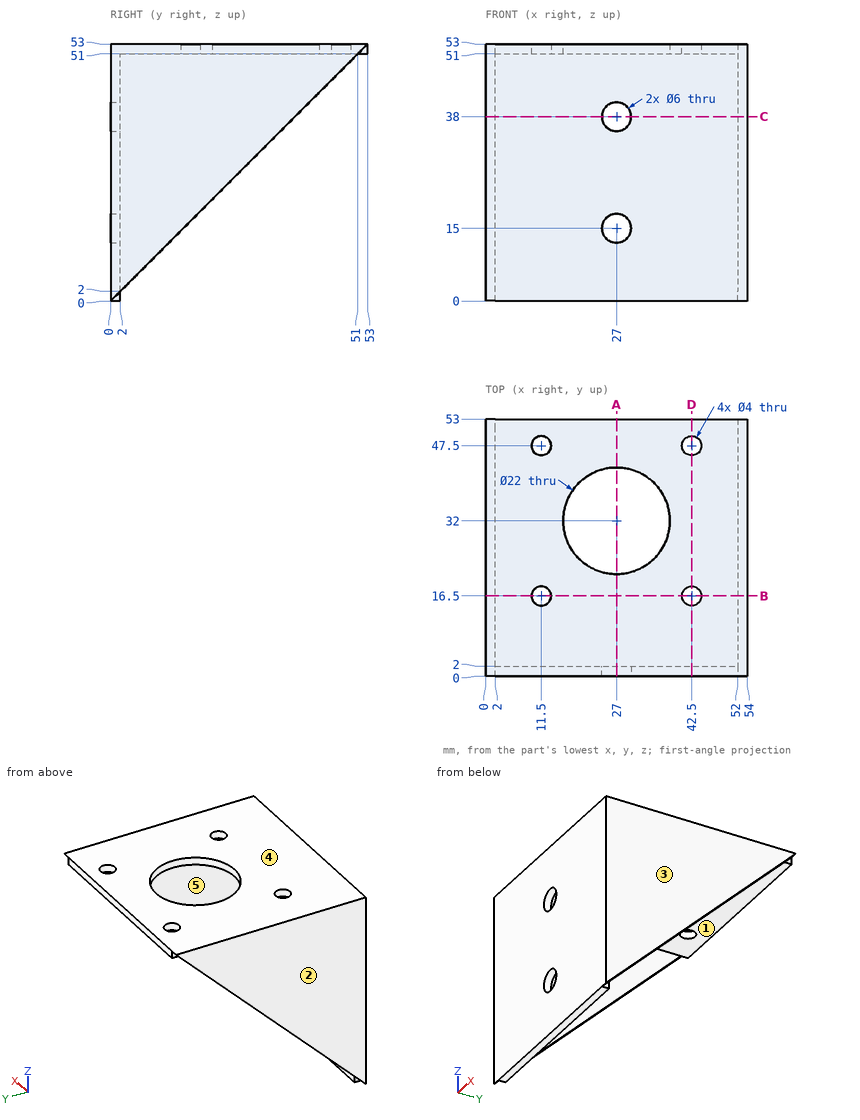
Check sheet for the drawn part. Datum: minimum x, y, z corner. Units: mm. A direction names the side the tool comes from. Round coordinates to 2 decimals unless told otherwise and drop trailing zeros. Loops run counter-clockwise (first coordinate to the right, second up) from the corner with the lowest first, then second, coordinate; pieces in that order, holes last. Notation, with made-up numbers: (69, 75.25) - (84, 75.25) arc R25 cw to (84, 107.25) - close; hole circle Ø5 at (74, 36.25). An arc over 180 degrees is marked (long way). Write item = value, one per line. Start each with the question number.
1. Section check A-A on x = 27. Enter the section's corners in (y, z).
2. Mould release check, pull along X, two halves, no side actions. Record for the marked faces 1, 2 and 3: released by +X, released by -X, zero draft, split by the parting line, or undercut.
3. Section check D-D on x = 42.5. Enter the section's corners in (y, z), then the cut area to 3 significant figures.
4. Depth check by flat-ended pin: pin 1 (4.5 mm diameter, centred on x = 11.5, y = 47.5, fed in from -Z); pin 2 (6 mm diameter, centred on x = 38, z = 40.5, fed in from +Y). Enter the tip coordinate at first touch or a pass-through.
5. Section check C-C on z = 38. Enter the section's corners in (x, y).
6. Section check B-B on y = 16.5. Enter the section's corners in (x, z).
7. Set-up check for the marked faces 4 and 5: record each of +Z, -Z, +X, -X, +Y, -Y from which the full face is reachable in a straight line by a thin tool's end or side.
8. Thickness scan on line 1 (Y direction, x = 11.5, z = 52.65); line 2 (Z direction, x = 27, y = 1.3); line 3 (X direction, y = 25, z = 34). Record the ranges inside material, lowest first.
Working result:
q1.outline = (0, 0) - (2, 0) - (2, 12) - (0, 12) - close; (0, 18) - (2, 18) - (2, 35) - (0, 35) - close; (0, 41) - (2, 41) - (2, 51) - (21, 51) - (21, 53) - (0, 53) - close; (43, 51) - (53, 51) - (53, 53) - (43, 53) - close
q2.face_1 = undercut
q2.face_2 = released by -X
q2.face_3 = released by +X
q3.outline = (0, 0) - (2, 0) - (2, 51) - (14.5, 51) - (14.5, 53) - (0, 53) - close; (18.5, 51) - (45.5, 51) - (45.5, 53) - (18.5, 53) - close; (49.5, 51) - (53, 51) - (53, 53) - (49.5, 53) - close
q3.area = 192 mm^2
q4.pin_1 = 51
q4.pin_2 = 2
q5.outline = (0, 0) - (24, 0) - (24, 2) - (2, 2) - (2, 38) - (0, 38) - close; (30, 0) - (54, 0) - (54, 38) - (52, 38) - (52, 2) - (30, 2) - close
q6.outline = (0, 16.5) - (2, 16.5) - (2, 51) - (9.5, 51) - (9.5, 53) - (0, 53) - close; (13.5, 51) - (40.5, 51) - (40.5, 53) - (13.5, 53) - close; (44.5, 51) - (52, 51) - (52, 16.5) - (54, 16.5) - (54, 53) - (44.5, 53) - close
q7.face_4 = +Z, +X, -X, +Y, -Y
q7.face_5 = -Z, +Y
q8.line_1 = 0 to 14.5, 18.5 to 45.5, 49.5 to 53
q8.line_2 = 0 to 12, 18 to 35, 41 to 53
q8.line_3 = 0 to 2, 52 to 54
